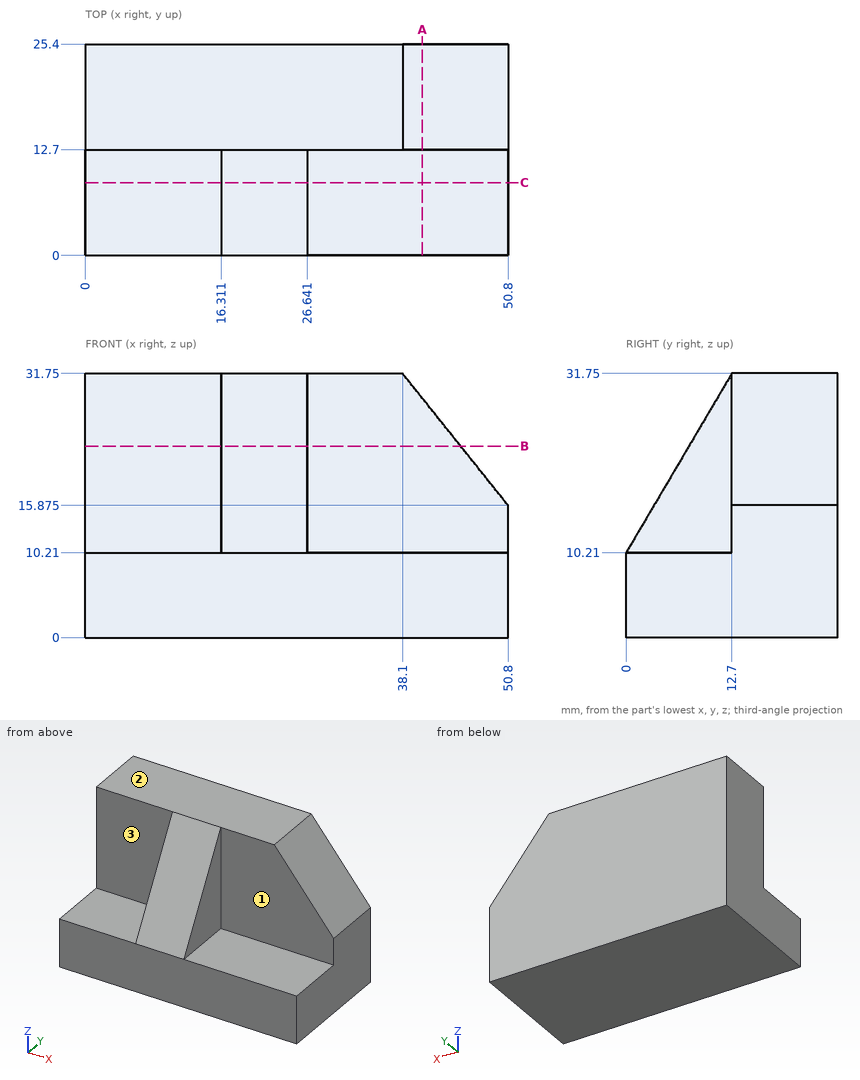
Design review of the part shown in the three views and the two pictorial views. Dimensions are in mm from the part's minimum x, y and z. A direction names the side the tool comes from. Give positions to 0.01 mm unless a question says otherwise; leave off trailing zeros. Write each loop counter-clockwise with the first axis right and the second up, starting at its lowest first coordinate (ties: lowest second). Pieces come first, ordered by that corner, then holes. Notation, with made-up numbers: M 68,-31 L 91,-31 A31 ccw 91,8 Z; hole C -23,54.5 d8. An arc over 180 degrees is marked long. Answer as CSV lines item,"result".
1. Consider section B-B, the plane z = 23. Write out the cut boundary in (x, y), then the cut area to 3 significant figures.
Findings:
outline,"M 0,12.7 L 16.31,12.7 L 16.31,7.54 L 26.64,7.54 L 26.64,12.7 L 45.1,12.7 L 45.1,25.4 L 0,25.4 Z"
area,"626 mm2"
2. For the marked faces 1, 2 and 3, list the 3-axis set-ups (+Z, -Z, +X, -X, +Y, -Y) from which the entire face can be reached by the end or side of a thin tool; tool diameter is ignored.
Findings:
face 1,"+Z, +X, -Y"
face 2,"+Z, +X, -X, +Y, -Y"
face 3,"+Z, -X, -Y"
3. Consider section C-C, the plane y = 8.75. Write out the cut boundary in (x, z).
Findings:
outline,"M 0,0 L 50.8,0 L 50.8,10.21 L 26.64,10.21 L 26.64,25.05 L 16.31,25.05 L 16.31,10.21 L 0,10.21 Z"
4. For pin 1 (14 mm diameter, centred on x = 41, y = 4, fed in from +Z); pin 2 (11 mm diameter, centred on x = 36, z = 20, fed in from -Y); pin 3 (4 mm diameter, centred on x = 41, y = 17.5, fed in from +Z) (1 decimal), all flat-tipped, find the tip position at first contact; note any pin that passes through.
Findings:
pin 1,"stops at z = 10.21"
pin 2,"stops at y = 12.7"
pin 3,"stops at z = 30.6"
5. Wall thickness on line 1 (Z direction, x = 14.5, y = 6.75); line 2 (Y direction, x = 9.5, z = 30); line 3 (X direction, y = 10.25, z = 12): over which ranges is each line inside the solid? List them lowest first.
Findings:
line 1,"z = 0 to 10.21"
line 2,"y = 12.7 to 25.4"
line 3,"x = 16.31 to 26.64"
6. Consider section A-A, the plane x = 40.5. Write out the cut boundary in (y, z).
Findings:
outline,"M 0,0 L 25.4,0 L 25.4,28.75 L 12.7,28.75 L 12.7,10.21 L 0,10.21 Z"
